Design review of the part built by this model. Coordinates are the model's own, in mm. A direction names the side the tool comes from. Coordinates: 2 decimals unless noted, no trailing zeros. Order: outer loops, then holes, each group sorted by start corner. A loop starts at its lowest first (then second) coordinate and runs counter-clockwise, first axis right, second up. Notation, with made-up numbers: M -25.5,15 L -10.5,15 A16 cw -10.5,33 Z; hole C 43.25,58 d6. An arc over 180 degrees is marked long. Answer in a Markdown table with one row per item.
from build123d import *

# Parameters (mm, degrees)
SKETCH1_W               = 33.703234699
SKETCH1_H               = 30.703234699
BOSS_EXTRUDE1_DEPTH     = 4
SKETCH1_3_W             = 33.703234699
SKETCH1_3_H             = 1.5
BOSS_EXTRUDE2_DEPTH     = 10
BOSS_EXTRUDE3_DEPTH     = 4
BOSS_EXTRUDE4_START     = 4
SKETCH4_R               = 2
BOSS_EXTRUDE4_DEPTH     = 4
CUT_EXTRUDE1_DEPTH      = 38
CUT_EXTRUDE1_DEPTH_BACK = 10
SKETCH11_W              = 20.703234699
SKETCH11_H              = 4


with BuildPart() as part:
    # Sketch1 → Boss-Extrude1 (new body)
    with BuildSketch(Plane(origin=(0, 0, 0), x_dir=(1, 0, 0), z_dir=(0, 1, 0))):
        with Locations((-16.851617349, -16.851617349)):
            Rectangle(SKETCH1_W, SKETCH1_H)
    extrude(amount=BOSS_EXTRUDE1_DEPTH)

    # Sketch1_3 → Boss-Extrude2 (add)
    with BuildSketch(Plane(origin=(0, 0, 0), x_dir=(1, 0, 0), z_dir=(0, 1, 0))):
        with Locations((-16.851617349, -32.953234699)):
            Rectangle(SKETCH1_3_W, SKETCH1_3_H)
        with Locations((-16.851617349, -0.75)):
            Rectangle(SKETCH1_3_W, SKETCH1_3_H)
    extrude(amount=BOSS_EXTRUDE2_DEPTH)

    # Sketch5 → Boss-Extrude3 (add)
    with BuildSketch(Plane(origin=(0, 0, 32.203234699), x_dir=(-1, 0, 0), z_dir=(0, 0, -1))):
        with BuildLine():
            ThreePointArc((6, 7), (5.414213562, 8.414213562), (4, 9))
            Line((4, 9), (4, 5))
            ThreePointArc((4, 5), (5.414213562, 5.585786438), (6, 7))
        make_face()
        with BuildLine():
            Line((4, 5), (4, 9))
            ThreePointArc((4, 9), (2, 7), (4, 5))
        make_face()
    extrude(amount=BOSS_EXTRUDE3_DEPTH)

    # Sketch4 → Boss-Extrude4 (add)
    with BuildSketch(Plane.XY.offset(1.5).offset(BOSS_EXTRUDE4_START)):
        with Locations(Location((-4, 7, 0), (0, 0, 180))):
            Circle(SKETCH4_R)
    extrude(amount=-BOSS_EXTRUDE4_DEPTH)

    # Sketch11 → Cut-Extrude1 (cut, two sides: drawn at the far end of the back side and taken through both)
    with BuildSketch(Plane(origin=(0, 0, 32.203234699), x_dir=(-1, 0, 0), z_dir=(0, 0, -1)).offset(-CUT_EXTRUDE1_DEPTH_BACK)):
        with BuildLine():
            Line((10, 9), (10, 5))
            ThreePointArc((10, 5), (8, 7), (10, 9))
        make_face()
        with Locations((20.35161735, 7)):
            Rectangle(SKETCH11_W, SKETCH11_H)
        with BuildLine():
            ThreePointArc((30.703234699, 5), (32.703234699, 7), (30.703234699, 9))
            Line((30.703234699, 9), (30.703234699, 5))
        make_face()
    extrude(amount=CUT_EXTRUDE1_DEPTH + CUT_EXTRUDE1_DEPTH_BACK, mode=Mode.SUBTRACT)


solid = part.part
(1) For line 1 along Y through (x, z) = (-4.5, 22); line 2 along Z through (x, y) = (-9, 4.25); line 3 along X through (y, z) = (5.25, 28.5), list the stretches that pass through material, from the lowest coordinate up. Write a range as from..to.
Return value:
| item | result |
|---|---|
| line 1 | y = 0..4 |
| line 2 | z = 0..1.5, 32.2..33.7 |
| line 3 | x = -4.97..-3.03 |
(2) Draft analysis for pull direction X (two halves, no side actions). For faces 1 (the flat face through (-33.703, 2, 17)), 2 (the flat face through (0, 2, 17)), 3 (the flat face through (-20, 9, 1)), 4 (the flat face through (-17, 10, 1)), state which applies: pulls with the +X half, pulls with the -X half, needs draft (parallel to the pull), parting line crosses it, or undercut.
Return value:
| item | result |
|---|---|
| face 1 | pulls with the -X half |
| face 2 | pulls with the +X half |
| face 3 | undercut |
| face 4 | needs draft |
(3) Add section C-C, the plane x = -9.5. Give the boundary of the cut face in (y, z), and give its area (3 significant figures).
Return value:
| item | result |
|---|---|
| outline | M 0,0 L 5.06,0 L 5.06,1.5 L 4,1.5 L 4,32.2 L 5.06,32.2 L 5.06,33.7 L 0,33.7 Z; M 8.94,0 L 10,0 L 10,1.5 L 8.94,1.5 Z; M 8.94,32.2 L 10,32.2 L 10,33.7 L 8.94,33.7 Z |
| area | 141 mm2 |
(4) Add section A-A, the plane z = 5. Give the boundary of the cut face in (x, y), and give its area (3 significant figures).
Return value:
| item | result |
|---|---|
| outline | M -33.7,0 L 0,0 L 0,4 L -33.7,4 Z; C -4,7 d4 |
| area | 147 mm2 |
(5) Add section B-B, the plane y = 7.5. Give the boundary of the cut face in (x, z).
Return value:
| item | result |
|---|---|
| outline | M -33.7,0 L -32.64,0 L -32.64,1.5 L -33.7,1.5 Z; M -33.7,32.2 L -32.64,32.2 L -32.64,33.7 L -33.7,33.7 Z; M -8.06,0 L 0,0 L 0,1.5 L -2.06,1.5 L -2.06,5.5 L -5.94,5.5 L -5.94,1.5 L -8.06,1.5 Z; M -8.06,32.2 L -5.94,32.2 L -5.94,28.2 L -2.06,28.2 L -2.06,32.2 L 0,32.2 L 0,33.7 L -8.06,33.7 Z |
(6) Insertion check: pin 1 Ø1.5 at (x, z) = (-12.5, 7.5) entering from +Y. The pin has a flat end and moves straight along its axis. Give the tip position at first contact, or say it passes through.
Return value:
| item | result |
|---|---|
| pin 1 | stops at y = 4 |
(7) Add section D-D, the plane y = 5.5. Give the boundary of the cut face in (x, z), and give its area (3 significant figures).
Return value:
| item | result |
|---|---|
| outline | M -33.7,0 L -32.03,0 L -32.03,1.5 L -33.7,1.5 Z; M -33.7,32.2 L -32.03,32.2 L -32.03,33.7 L -33.7,33.7 Z; M -8.68,0 L 0,0 L 0,1.5 L -2.68,1.5 L -2.68,5.5 L -5.32,5.5 L -5.32,1.5 L -8.68,1.5 Z; M -8.68,32.2 L -5.32,32.2 L -5.32,28.2 L -2.68,28.2 L -2.68,32.2 L 0,32.2 L 0,33.7 L -8.68,33.7 Z |
| area | 52.2 mm2 |
(8) For faces 5 (the cylindrical face through (-8, 7, 1)), 6 (the flat face through (-17, 4, 0)), 7 (the flat face through (-4, 7, 28.203)), list the 3-axis set-ups (+Z, -Z, +X, -X, +Y, -Y) from which the entire face can be reached by the end or side of a thin tool; tool diameter is ignored.
Return value:
| item | result |
|---|---|
| face 5 | +Z, -Z |
| face 6 | -Z, +X, -X, +Y, -Y |
| face 7 | +X, -X, +Y |
